CAD build for the part. Positions are in the model's coordinates, mm. Face numbers are marked on the shaded views. A direction names the side the tool comes from. Give positions to 0.01 mm unless a question says otherwise; leave off trailing zeros. Write each loop counter-clockwise with the first axis right and the second up, starting at its lowest first coordinate (ties: lowest second). Pieces come first, ordered by that corner, then holes. Notation, with made-up numbers: (-7, 80) - (2, 80) arc R10 ccw to (2, 94) - close; hole circle Ø4 at (-12, 59). An arc over 180 degrees is marked (long way). Answer as a JSON object with one key per item and string values.
from build123d import *

# Parameters (mm, degrees)
EXTRUDE_1_DEPTH     = 30
CUT_EXTRUDE_1_DEPTH = 21
SKETCH_3_R          = 1.5
CUT_EXTRUDE_2_DEPTH = 31


with BuildPart() as part:
    # Эскиз1 → Вытянуть-Тонкостенный1 (new body)
    with BuildSketch(Plane(origin=(0, 0, 0), x_dir=(0, 0, -1), z_dir=(1, 0, 0))):
        Polygon((0, 0), (0, 30), (20, 30), (20, 0), (18, 0), (18, 28), (2, 28), (2, 0), align=None)
    extrude(amount=EXTRUDE_1_DEPTH)

    # Эскиз2 → Вырез-Вытянуть1 (cut, through all)
    with BuildSketch(Plane.XY):
        Polygon((0, 0), (30, 20), (30, 0), align=None)
    extrude(amount=-CUT_EXTRUDE_1_DEPTH, mode=Mode.SUBTRACT)

    # Эскиз3 → Вырез-Вытянуть2 (cut, through all)
    with BuildSketch(Plane(origin=(0, 30, 0), x_dir=(1, 0, 0), z_dir=(0, 1, 0))):
        with Locations((18, 10)):
            Circle(SKETCH_3_R)
    extrude(amount=-CUT_EXTRUDE_2_DEPTH, mode=Mode.SUBTRACT)


solid = part.part
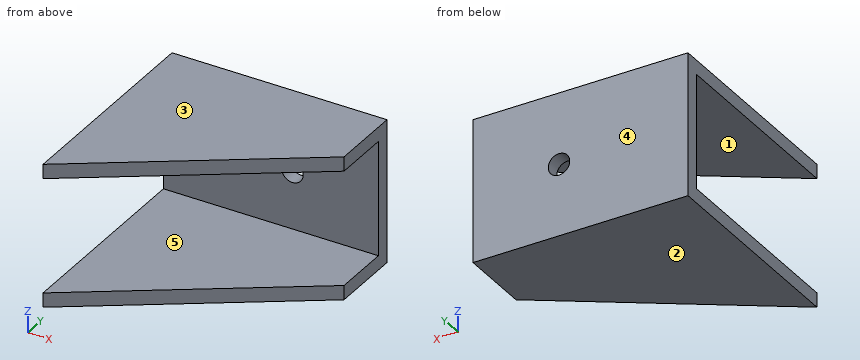
(1) Flat gauge pin, fed straight in: P1, Ø5, axis at x = 21, z = -9.5, coming from the -Y side. Where does the tip first touch, or does it go through?
Answer key:
{"P1": "stops at y = 28"}
(2) Saw through at A-A, the plane y = 20.5. Give the cut face in (x, z), and give its area (3 significant figures).
Answer key:
{"outline": "(0, -20) - (30, -20) - (30, -18) - (0, -18) - close; (0, -2) - (30, -2) - (30, 0) - (0, 0) - close", "area": "120 mm²"}
(3) Saw through at B-B, the plane x = 18. Give the cut face in (y, z).
Answer key:
{"outline": "(12, -20) - (30, -20) - (30, -11.5) - (28, -11.5) - (28, -18) - (12, -18) - close; (12, -2) - (28, -2) - (28, -8.5) - (30, -8.5) - (30, 0) - (12, 0) - close"}
(4) Saw through at D-D, the plane z = -12.5. Give the cut face in (x, y).
Answer key:
{"outline": "(0, 28) - (30, 28) - (30, 30) - (0, 30) - close"}
(5) Saw through at C-C, the plane z = -10. Give the cut face in (x, y), and give its area (3 significant figures).
Answer key:
{"outline": "(0, 28) - (16.5, 28) - (16.5, 30) - (0, 30) - close; (19.5, 28) - (30, 28) - (30, 30) - (19.5, 30) - close", "area": "54.0 mm²"}
(6) Pull direction Z, two halves, no side cores. Call the marked faces 3, 4 and 5: pulls with the +Z half, pulls with the -Z half, needs draft (parallel to the pull), parting line crosses it, or undercut.
Answer key:
{"face 3": "pulls with the +Z half", "face 4": "needs draft", "face 5": "undercut"}
(7) 3-axis set-ups, long thin cutter, end or side, ignore diameter. For the marked faces 1 and 2: which of +Z, -Z, +X, -X, +Y, -Y reach the whole face in a straight line?
Answer key:
{"face 1": "+X, -X, -Y", "face 2": "-Z, +X, -X, +Y, -Y"}
(8) Probe L1, parallel to Z at x = 18, y = 29.6; L2, parallel to Z at x = 3, y = 9.25; L3, parallel to X at y = 28.55, z = -10. List the from-to ranges inside material, lowest first. Write a range as [from, to].
Answer key:
{"L1": "z = [-20, -11.5], [-8.5, 0]", "L2": "z = [-20, -18], [-2, 0]", "L3": "x = [0, 16.5], [19.5, 30]"}
